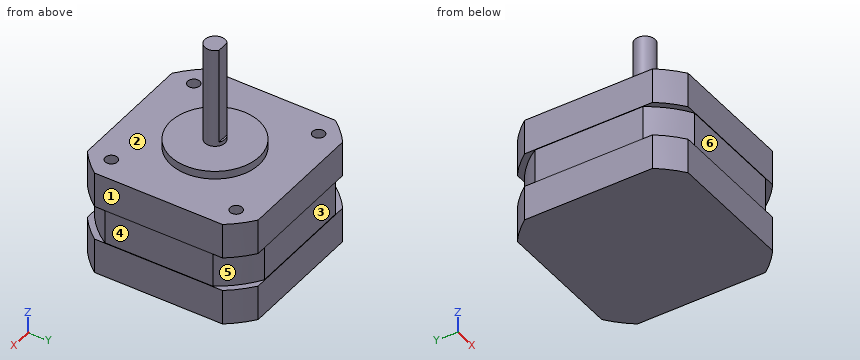
from build123d import *

# Parameters (mm, degrees)
SKETCH1_R                       = 2.5
BOSS_EXTRUDE1_DEPTH             = 27
SKETCH2_R                       = 11
BOSS_EXTRUDE2_DEPTH             = 2
SKETCH3_W                       = 42.418
SKETCH3_H                       = 42.418
BOSS_EXTRUDE3_DEPTH             = 26
CUT_EXTRUDE1_DEPTH              = 54
M3X0_5_TAPPED_HOLE1_D           = 2.5
M3X0_5_TAPPED_HOLE1_DEPTH       = 7.5
M3X0_5_TAPPED_HOLE1_CBORE_D     = 3
M3X0_5_TAPPED_HOLE1_CBORE_DEPTH = 6
M3X0_5_TAPPED_HOLE1_TIP         = 0.751075774
CUT_EXTRUDE2_DEPTH              = 24
CUT_EXTRUDE3_DEPTH              = 4.25
CUT_EXTRUDE3_DEPTH_BACK         = 4.25


with BuildPart() as part:
    # Sketch1 → Boss-Extrude1 (new body)
    with BuildSketch(Plane.XY):
        Circle(SKETCH1_R)
    extrude(amount=BOSS_EXTRUDE1_DEPTH)

    # Sketch2 → Boss-Extrude2 (add)
    with BuildSketch(Plane(origin=(0, 0, 0), x_dir=(-1, 0, 0), z_dir=(0, 0, -1))):
        Circle(SKETCH2_R)
    extrude(amount=-BOSS_EXTRUDE2_DEPTH)

    # Sketch3 → Boss-Extrude3 (add)
    with BuildSketch(Plane(origin=(0, 0, 0), x_dir=(-1, 0, 0), z_dir=(0, 0, -1))):
        Rectangle(SKETCH3_W, SKETCH3_H)
    extrude(amount=BOSS_EXTRUDE3_DEPTH)

    # Sketch4 → Cut-Extrude1 (cut, through all)
    with BuildSketch(Plane(origin=(0, 0, -26), x_dir=(-1, 0, 0), z_dir=(0, 0, -1))):
        with BuildLine():
            Line((-21.209, -15.887992919), (-21.209, -21.209))
            Line((-21.209, -21.209), (-15.887992919, -21.209))
            ThreePointArc((-15.887992919, -21.209), (-18.738329701, -18.738329701), (-21.209, -15.887992919))
        make_face()
        with BuildLine():
            Line((15.887992919, -21.209), (21.209, -21.209))
            Line((21.209, -21.209), (21.209, -15.887992919))
            ThreePointArc((21.209, -15.887992919), (18.738329701, -18.738329701), (15.887992919, -21.209))
        make_face()
        with BuildLine():
            Line((21.209, 15.887992919), (21.209, 21.209))
            Line((21.209, 21.209), (15.887992919, 21.209))
            ThreePointArc((15.887992919, 21.209), (18.738329701, 18.738329701), (21.209, 15.887992919))
        make_face()
        with BuildLine():
            Line((-15.887992919, 21.209), (-21.209, 21.209))
            Line((-21.209, 21.209), (-21.209, 15.887992919))
            ThreePointArc((-21.209, 15.887992919), (-18.738329701, 18.738329701), (-15.887992919, 21.209))
        make_face()
    extrude(amount=-CUT_EXTRUDE1_DEPTH, mode=Mode.SUBTRACT)

    # M3x0.5 Tapped Hole1
    with Locations(Plane.XY):
        with Locations((-15.5, 15.5), (-15.5, -15.5), (15.5, -15.5), (15.5, 15.5)):
            CounterBoreHole(M3X0_5_TAPPED_HOLE1_D / 2, M3X0_5_TAPPED_HOLE1_CBORE_D / 2, M3X0_5_TAPPED_HOLE1_CBORE_DEPTH, depth=M3X0_5_TAPPED_HOLE1_DEPTH)
            with Locations((0, 0, -(M3X0_5_TAPPED_HOLE1_DEPTH + M3X0_5_TAPPED_HOLE1_TIP / 2))):  # 118° drill point
                Cone(0, M3X0_5_TAPPED_HOLE1_D / 2, M3X0_5_TAPPED_HOLE1_TIP, mode=Mode.SUBTRACT)

    # Sketch7 → Cut-Extrude2 (cut)
    with BuildSketch(Plane.XY.offset(27)):
        with BuildLine():
            Line((-1.5, 2), (1.5, 2))
            ThreePointArc((1.5, 2), (0, 2.5), (-1.5, 2))
        make_face()
    extrude(amount=-CUT_EXTRUDE2_DEPTH, mode=Mode.SUBTRACT)

    # Sketch8 → Cut-Extrude3 (cut, two sides)
    with BuildSketch(Plane.XY.offset(-13)) as cut_extrude3_sk:
        with BuildLine():
            Line((15.887992919, 21.209), (-15.887992919, 21.209))
            ThreePointArc((-15.887992919, 21.209), (-18.738329701, 18.738329701), (-21.209, 15.887992919))
            Line((-21.209, 15.887992919), (-21.209, -15.887992919))
            ThreePointArc((-21.209, -15.887992919), (-18.738329701, -18.738329701), (-15.887992919, -21.209))
            Line((-15.887992919, -21.209), (15.887992919, -21.209))
            ThreePointArc((15.887992919, -21.209), (18.738329701, -18.738329701), (21.209, -15.887992919))
            Line((21.209, -15.887992919), (21.209, 15.887992919))
            ThreePointArc((21.209, 15.887992919), (18.738329701, 18.738329701), (15.887992919, 21.209))
        make_face()
        with BuildLine():
            Line((-13.394406258, 21.109), (13.394406258, 21.109))
            ThreePointArc((13.394406258, 21.109), (17.67766953, 17.67766953), (21.109, 13.394406258))
            Line((21.109, 13.394406258), (21.109, -13.394406258))
            ThreePointArc((21.109, -13.394406258), (17.67766953, -17.67766953), (13.394406258, -21.109))
            Line((13.394406258, -21.109), (-13.394406258, -21.109))
            ThreePointArc((-13.394406258, -21.109), (-17.67766953, -17.67766953), (-21.109, -13.394406258))
            Line((-21.109, -13.394406258), (-21.109, 13.394406258))
            ThreePointArc((-21.109, 13.394406258), (-17.67766953, 17.67766953), (-13.394406258, 21.109))
        make_face(mode=Mode.SUBTRACT)
    extrude(amount=CUT_EXTRUDE3_DEPTH, mode=Mode.SUBTRACT)
    extrude(cut_extrude3_sk.sketch, amount=-CUT_EXTRUDE3_DEPTH_BACK, mode=Mode.SUBTRACT)


solid = part.part
Design review of the part built by this model. Coordinates are the model's own, in mm. Face numbers are marked on the shaded views. A direction names the side the tool comes from. Give positions to 0.01 mm unless a question says otherwise; leave off trailing zeros. Write each loop counter-clockwise with the first axis right and the second up, starting at its lowest first coordinate (ties: lowest second). Pieces come first, ordered by that corner, then holes. Notation, with made-up numbers: M -35,70 L 7,70 A19 ccw 7,87 Z; hole C 8.5,26 d2. An arc over 180 degrees is marked long. Return JSON: item names as keys, results as strings. Group by question number.
Item 1: Clearance check with flat-ended pins moving along their axes: pin 1 Ø1.5 at (x, y) = (-15.5, 15.5) entering from +Z; pin 2 Ø0.9 at (x, y) = (-15, -15) entering from +Z; pin 3 Ø3 at (x, z) = (-0.5, 7) entering from +Y. State where each tip first meets the part, or that it passes through.
Item 2: Take a section at A-A (z = -20.5). Give the boundary of the cut face in (x, y), plus the area to 3 significant figures.
Item 3: The part is to be moulded in two halves that separate along Z. For the marked faces 1, 2 and 3, say which applies: pulls with the +Z half, pulls with the -Z half, needs draft (parallel to the pull), parting line crosses it, or undercut.
Item 4: Take a section at B-B (x = -12.5). Give the boundary of the cut face in (y, z), plus the area to 3 significant figures.
Item 5: Take a section at D-D (x = 0). Give the boundary of the cut face in (y, z).
Item 6: Tool access review of the marked faces 4, 5 and 6: name each direction out of +Z, -Z, +X, -X, +Y, -Y from which nothing blocks a thin tool from reaching the whole face with its end or side.
Item 7: Wall thickness on line 1 along Y through (x, z) = (15.5, -3.2); line 2 along X through (y, z) = (-15.5, -7.1): over which ranges is each line inside the solid? List them lowest first.
Return value:
{
 "1": {"pin 1": "stops at z = -7.8", "pin 2": "stops at z = -7.56", "pin 3": "stops at y = 2"},
 "2": {"outline": "M -21.21,-15.89 A26.5 ccw -15.89,-21.21 L 15.89,-21.21 A26.5 ccw 21.21,-15.89 L 21.21,15.89 A26.5 ccw 15.89,21.21 L -15.89,21.21 A26.5 ccw -21.21,15.89 Z", "area": "1,750 mm2"},
 "3": {"face 1": "needs draft", "face 2": "pulls with the +Z half", "face 3": "undercut"},
 "4": {"outline": "M -21.21,-26 L 21.21,-26 L 21.21,-17.25 L 21.11,-17.25 L 21.11,-8.75 L 21.21,-8.75 L 21.21,0 L -21.21,0 L -21.21,-8.75 L -21.11,-8.75 L -21.11,-17.25 L -21.21,-17.25 Z", "area": "1,100 mm2"},
 "5": {"outline": "M -21.21,-26 L 21.21,-26 L 21.21,-17.25 L 21.11,-17.25 L 21.11,-8.75 L 21.21,-8.75 L 21.21,0 L 11,0 L 11,2 L 2.5,2 L 2.5,3 L 2,3 L 2,27 L -2.5,27 L -2.5,2 L -11,2 L -11,0 L -21.21,0 L -21.21,-8.75 L -21.11,-8.75 L -21.11,-17.25 L -21.21,-17.25 Z"},
 "6": {"face 4": "+X, +Y, -Y", "face 5": "+X, +Y", "face 6": "+X, -X, -Y"},
 "7": {"line 1": "y = -21.21 to -17, -14 to 14, 17 to 21.21", "line 2": "x = -21.21 to -16.75, -14.25 to 14.25, 16.75 to 21.21"}
}
